from build123d import *

# Parameters (mm, degrees)
ESQUISSE1_R             = 29
BOSS_EXTRU_1_DEPTH      = 20
ESQUISSE2_R             = 40
BOSS_EXTRU_2_DEPTH      = 10
CHANFREIN1_SIZE         = 5
ESQUISSE3_R             = 2
ENL_V_MAT_EXTRU_1_DEPTH = 30
ESQUISSE4_W             = 5
ESQUISSE4_H             = 7
BOSS_EXTRU_4_DEPTH      = 10


with BuildPart() as part:
    # Esquisse1 → Boss.-Extru.1 (new body)
    with BuildSketch(Plane.XY):
        Circle(ESQUISSE1_R)
    extrude(amount=BOSS_EXTRU_1_DEPTH)

    # Esquisse2 → Boss.-Extru.2 (add)
    with BuildSketch(Plane.XY.offset(20)):
        Circle(ESQUISSE2_R)
    extrude(amount=BOSS_EXTRU_2_DEPTH)

    # Chanfrein1
    chanfrein1_edges = [part.edges().sort_by_distance(p)[0] for p in [
        (-29, 0, 0),
    ]]
    chamfer(chanfrein1_edges, length=CHANFREIN1_SIZE)

    # Esquisse3 → Enlèv. mat.-Extru.1 (cut)
    with BuildSketch(Plane.XY.offset(30)):
        Circle(ESQUISSE3_R)
    extrude(amount=-ENL_V_MAT_EXTRU_1_DEPTH, mode=Mode.SUBTRACT)

    # Esquisse4 → Boss.-Extru.4 (add)
    with BuildSketch(Plane(origin=(0, 0, 0), x_dir=(-1, 0, 0), z_dir=(0, 0, -1))):
        with Locations((0, 6.5)):
            Rectangle(ESQUISSE4_W, ESQUISSE4_H)
        with Locations((0, -6.5)):
            Rectangle(ESQUISSE4_W, ESQUISSE4_H)
    extrude(amount=BOSS_EXTRU_4_DEPTH)


solid = part.part
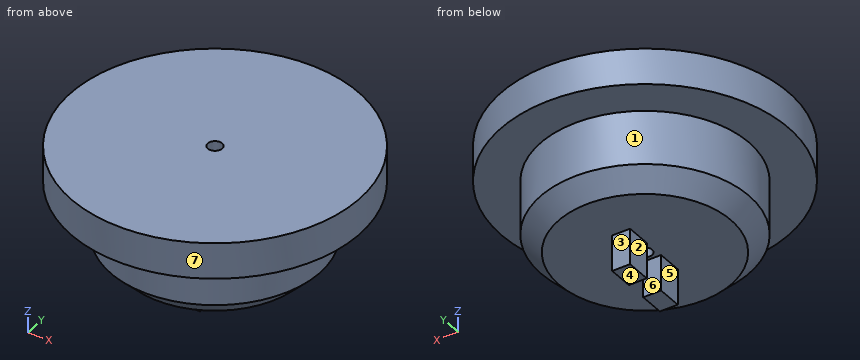
Check sheet for the modelled part. Datum: model origin and axes. Units: mm. Face numbers are marked on the shaded views. A direction names the side the tool comes from. Give positions to 0.01 mm unless a question says otherwise; leave off trailing zeros. Loops run counter-clockwise (first coordinate to the right, second up) from the corner with the lowest first, then second, coordinate; pieces in that order, holes last. Notation, with made-up numbers: M 55.5,-16 L 81.5,-16 A14 ccw 81.5,-9 Z; hole C 83,-23 d1. An arc over 180 degrees is marked long. Answer as a JSON object with one key per item and string values. Group by question number.
Q1. Go/stop test with flat-tipped pins: P1, Ø5.5, axis at y = -6, z = -6, coming from the +X side; P2, Ø1.5, axis at x = -1, z = -3.5, coming from the +Y side; P3, Ø24, axis at x = -10.5, y = -1, coming from the -Z side; P4, Ø3, axis at x = -9.5, z = 23, coming from the -Y side. Record where each tip stops, or that it passes through.
Q2. Cross-section at D-D on z = 11.5. Record the cut outline in (x, y).
Q3. Cross-section at B-B on z = -5. Record the cut outline in (x, y).
Q4. Cross-section at C-C on y = 0. Record the cut outline in (x, z).
Q5. Cross-section at A-A on x = 0. Record the cut outline in (y, z).
Q6. Access from +Z, -Z, +X, -X, +Y, -Y to the whole of each face (thin tool, end or side, straight path). Record for the marked faces 1, 2, 3 and 4.
Q7. Release check for a two-part mould opening along Y. For the marked faces 5, 6 and 7 record: released by +Y, released by -Y, zero draft, split by the parting line, or undercut.
Q8. Material ranges on line 1 along Y through (x, z) = (0, 18.5); line 2 along Y through (x, z) = (0, 20.75); line 3 along Z through (x, y) = (-12.5, -4), recorded low to high. Write a range as [from, to].
Evaluation:
{
 "1": {"P1": "stops at x = 2.5", "P2": "stops at y = 10", "P3": "stops at z = -10", "P4": "stops at y = -39.19"},
 "2": {"outline": "C 0,0 d58; hole C 0,0 d4"},
 "3": {"outline": "M -2.5,-10 L 2.5,-10 L 2.5,-3 L -2.5,-3 Z; M -2.5,3 L 2.5,3 L 2.5,10 L -2.5,10 Z"},
 "4": {"outline": "M -40,20 L -29,20 L -29,5 L -24,0 L -2,0 L -2,30 L -40,30 Z; M 2,0 L 24,0 L 29,5 L 29,20 L 40,20 L 40,30 L 2,30 Z"},
 "5": {"outline": "M -40,20 L -29,20 L -29,5 L -24,0 L -10,0 L -10,-10 L -3,-10 L -3,0 L -2,0 L -2,30 L -40,30 Z; M 2,0 L 3,0 L 3,-10 L 10,-10 L 10,0 L 24,0 L 29,5 L 29,20 L 40,20 L 40,30 L 2,30 Z"},
 "6": {"face 1": "-Z", "face 2": "-Z, -X, +Y, -Y", "face 3": "-Z, +X, -X, +Y", "face 4": "-Z, +X, -X, +Y, -Y"},
 "7": {"face 5": "zero draft", "face 6": "undercut", "face 7": "split by the parting line"},
 "8": {"line 1": "y = [-29, -2], [2, 29]", "line 2": "y = [-40, -2], [2, 40]", "line 3": "z = [0, 30]"}
}
